from build123d import *

# Parameters (mm, degrees)
SKETCH1_W                           = 96.210678118
SKETCH1_H                           = 96.210678118
SKETCH1_R                           = 4.25
BODY_EXTRUSION_AND_BOLT_HOLES_DEPTH = 22.5
SKETCH3_R                           = 10
ENTRANCE_DEPTH                      = 22.5
SKETCH5_R                           = 2.5
CUT_EXTRUDE1_DEPTH                  = 100


with BuildPart() as part:
    # Sketch1 → body extrusion and bolt holes (new body)
    with BuildSketch(Plane(origin=(0, 0, 0), x_dir=(1, 0, 0), z_dir=(0, 1, 0))):
        Rectangle(SKETCH1_W, SKETCH1_H)
        with Locations(Location((-35.355339059, 35.355339059, 0), (0, 0, 90))):
            Circle(SKETCH1_R, mode=Mode.SUBTRACT)
        with Locations(Location((35.355339059, 35.355339059, 0), (0, 0, 90))):
            Circle(SKETCH1_R, mode=Mode.SUBTRACT)
        with Locations(Location((35.355339059, -35.355339059, 0), (0, 0, 90))):
            Circle(SKETCH1_R, mode=Mode.SUBTRACT)
        with Locations(Location((-35.355339059, -35.355339059, 0), (0, 0, 90))):
            Circle(SKETCH1_R, mode=Mode.SUBTRACT)
    extrude(amount=BODY_EXTRUSION_AND_BOLT_HOLES_DEPTH)

    # Sketch2 → main chamber (revolve, cut)
    with BuildSketch(Plane.XY):
        Polygon((0, 0), (0, 14.5), (22.725, 6.5), (22.725, 0), align=None)
    revolve(axis=Axis((0, 0, 0), (0, 1, 0)), mode=Mode.SUBTRACT)

    # Sketch3 → entrance (cut)
    with BuildSketch(Plane(origin=(0, 22.5, 0), x_dir=(1, 0, 0), z_dir=(0, 1, 0))):
        with Locations(Location((0, 0, 0), (0, 0, 270))):
            Circle(SKETCH3_R)
    extrude(amount=-ENTRANCE_DEPTH, mode=Mode.SUBTRACT)

    # Sketch5 → Cut-Extrude1 (cut)
    with BuildSketch(Plane(origin=(0, 0, 0), x_dir=(0, 0, -1), z_dir=(1, 0, 0))):
        with Locations((-20.225, 4)):
            Circle(SKETCH5_R)
    extrude(amount=-CUT_EXTRUDE1_DEPTH, mode=Mode.SUBTRACT)


solid = part.part
The listing builds one solid part. Answer for the finished solid, in the listing's coordinates (mm). A direction names the side the tool comes from. Give positions to 0.01 mm unless a question says otherwise; leave off trailing zeros. Loops run counter-clockwise (first coordinate to the right, second up) from the corner with the lowest first, then second, coordinate; pieces in that order, holes last. Notation, with made-up numbers: (46.25, 68) - (60.25, 68) arc R15 cw to (60.25, 77) - close; hole circle Ø7 at (-12, 50). An arc over 180 degrees is marked (long way). Answer as a JSON object with one key per item and string values.
1. A cutting plane is placed at D-D (y = 2.75). Write down the section's boundary in (x, z) (3 decimals).
Determined:
{"outline": "(-48.105, -48.105) - (48.105, -48.105) - (48.105, 48.105) - (-48.105, 48.105) - (-48.105, 22.39) - (-3.887, 22.39) arc R22.725 cw (long way) to (-13.794, 18.06) - (-48.105, 18.06) - close; hole circle Ø8.5 at (-35.355, -35.355); hole circle Ø8.5 at (-35.355, 35.355); hole circle Ø8.5 at (35.355, -35.355); hole circle Ø8.5 at (35.355, 35.355)"}
2. A cutting plane is placed at C-C (y = 14.75). Write down the section's boundary in (x, z).
Determined:
{"outline": "(-48.11, -48.11) - (48.11, -48.11) - (48.11, 48.11) - (-48.11, 48.11) - close; hole circle Ø8.5 at (-35.36, -35.36); hole circle Ø8.5 at (-35.36, 35.36); hole circle Ø20 at (0, 0); hole circle Ø8.5 at (35.36, -35.36); hole circle Ø8.5 at (35.36, 35.36)"}
3. Find the intervals of material crossed by L1, parallel to Z at x = 35, y = 10.75; L2, parallel to X at y = 2.75, z = 32; L3, parallel to X at y = 5.5, z = -34.5, in increasing order. Write a range as [from, to].
Determined:
{"L1": "[-48.11, -39.59], [-31.12, 31.12], [39.59, 48.11]", "L2": "[-48.11, -37.96], [-32.75, 32.75], [37.96, 48.11]", "L3": "[-48.11, -39.52], [-31.19, 31.19], [39.52, 48.11]"}
4. A cutting plane is placed at A-A (z = 0). Write down the section's boundary in (x, y) (3 decimals).
Determined:
{"outline": "(-48.105, 0) - (-22.725, 0) - (-22.725, 6.5) - (-10, 10.98) - (-10, 22.5) - (-48.105, 22.5) - close; (10, 10.98) - (22.725, 6.5) - (22.725, 0) - (48.105, 0) - (48.105, 22.5) - (10, 22.5) - close"}
5. A cutting plane is placed at B-B (x = 38.5). Write down the section's boundary in (y, z).
Determined:
{"outline": "(0, -48.11) - (22.5, -48.11) - (22.5, -38.21) - (0, -38.21) - close; (0, -32.5) - (22.5, -32.5) - (22.5, 32.5) - (0, 32.5) - close; (0, 38.21) - (22.5, 38.21) - (22.5, 48.11) - (0, 48.11) - close"}
6. For a pull along Y with two mould halves and no side action, classify faces 3 (the flat face through (-1, 22.5, -11)), 4 (the cylindrical face through (-29.061, 4.11, 22.723)), 5 (the cylindrical face through (-38.2, 11.1, -32.2)), 6 (the conical face through (-2.34, 10.7, 10.54)) as pulls with the +Y half, pulls with the -Y half, needs draft (parallel to the pull), parting line crosses it, or undercut.
Determined:
{"face 3": "pulls with the +Y half", "face 4": "undercut", "face 5": "needs draft", "face 6": "pulls with the -Y half"}
7. For faces 1 (the cylindrical face through (12.22, 3.2, -19.16)), 2 (the cylindrical face through (35.17, 11.09, 39.6)), determine the directions among +Z, -Z, +X, -X, +Y, -Y from which every point of the face is accessible in a straight line to the end or side of a thin tool.
Determined:
{"face 1": "-Y", "face 2": "+Y, -Y"}
